Autodesk Inventor part; units mm, degrees
ref_plane "YZ Plane" through (0, 0, 0) normal (1, 0, 0) x (0, 1, 0)
ref_plane "XZ Plane" through (0, 0, 0) normal (0, 1, 0) x (-1, 0, 0)
ref_plane "XY Plane" through (0, 0, 0) normal (0, 0, 1) x (1, 0, 0)
sketch "Sketch1" plane through (0, 0, 0) normal (0, 0, 1) x (1, 0, 0)
  line L0 (0, 0) -> (45, 0)
  line L1 (45, 0) -> (45, 45)
  line L2 (45, 45) -> (0, 45)
  line L3 (0, 45) -> (0, 0)
  dimension "d0" = 45
  dimension "d1" = 45
extrude "Extrusion1" add sketch "Sketch1" along normal blind 50
fillet "Fillet1" radius 5 4 edges at (45, 45, 25) (0, 45, 25) (45, 0, 25) (0, 0, 25)
sketch "Sketch2" plane through (0, 0, 0) normal (0, 0, -1) x (-1, 0, 0)
  line L0 (-45, 5) -> (-45, 40)
  line L1 (-45, 22.5) -> (-22.5, 22.5)
  circle A0 centre (-22.5, 22.5) radius 7.5
  point P0 (0, 0)
  dimension "d5" = 22.5
  dimension "d6" = 15
extrude "Extrusion2" cut sketch "Sketch2" against normal blind 20
sketch "Sketch3" plane through (0, 0, 50) normal (0, 0, 1) x (1, 0, 0)
  line L0 (0, 0) -> (3.5, 0)
  line L1 (5, 0) -> (40, 0)
  line L2 (3.5, 0) -> (3.5, 12)
  line L3 (3.5, 12) -> (41.5, 12)
  line L4 (41.5, 12) -> (41.5, 33)
  line L5 (41.5, 33) -> (3.5, 33)
  line L6 (3.5, 33) -> (3.5, 12)
  dimension "d11" = 3.5
  dimension "d12" = 12
  dimension "d13" = 38
  dimension "d14" = 21
extrude "Extrusion3" cut sketch "Sketch3" against normal blind 12
sketch "Sketch4" plane through (0, 0, 38) normal (0, 0, 1) x (1, 0, 0)
  line L0 (3.5, 12) -> (3.5, 33)
  line L1 (3.5, 22.5) -> (29.5, 22.5)
  line L2 (29.5, 22.5) -> (33.5, 22.5)
  line L3 (3.5, 33) -> (41.5, 33)
  line L4 (30.5, 33) -> (37.7775, 33)
  line L5 (37.7775, 33) -> (37.7775, 12)
  line L6 (37.7775, 12) -> (30.5, 12)
  line L7 (30.5, 12) -> (30.5, 33)
  point P0 (0, 0)
  dimension "d20" = 26
  dimension "d21" = 4
extrude "Extrusion4" cut sketch "Sketch4" against normal blind 7 contours L3 L5 L6 L7
sketch "Sketch5" plane through (0, 0, 38) normal (0, 0, 1) x (1, 0, 0)
  circle A0 centre (9.0685, 22.5) radius 3.5
  point P0 (0, 0)
  dimension "d24" = 7
extrude "Extrusion5" cut sketch "Sketch5" against normal blind 40
sketch "Sketch6" plane through (0, 0, 50) normal (0, 0, 1) x (1, 0, 0)
  line L0 (3.5, 33) -> (30.5, 33)
  line L1 (3.5, 33) -> (0, 33)
  line L2 (0, 40) -> (0, 5)
  line L3 (3.5, 11.9982) -> (0, 11.9982)
  line L4 (0, 33) -> (3.5, 33)
  line L5 (3.5, 33) -> (3.5, 11.9982)
  line L6 (3.5, 11.9982) -> (0, 11.9982)
  line L7 (0, 11.9982) -> (0, 33)
  point P0 (0, 0)
extrude "Extrusion6" add sketch "Sketch6" along normal blind 30
fillet "Fillet2" radius 10.5 2 edges at (1.75, 33, 80) (1.75, 11.9982, 80)
sketch "Sketch7" plane through (0, 5, 0) normal (-1, 0, 0) x (0, 0, 1)
  arc A0 (80, 17.5) -> (69.5, 28) centre (69.5, 17.5) ccw
  circle A1 centre (69.5, 17.5) radius 1.5
  point P0 (0, -5)
  dimension "d30" = 3
extrude "Extrusion7" cut sketch "Sketch7" against normal blind 30
properties part number "Motor holder"
The listing builds one solid part. Answer for the finished solid, in the listing's coordinates (mm). A direction names the side the tool comes from. Round coordinates to 2 decimals unless told otherwise and drop trailing zeros. Loops run counter-clockwise (first coordinate to the right, second up) from the corner with the lowest first, then second, coordinate; pieces in that order, holes last. Notation, with made-up numbers: M 70.25,3.5 L 119.25,3.5 A18 cw 119.25,35.5 Z; hole C 21.25,13 d4. An arc over 180 degrees is marked long. Return JSON: item names as keys, results as strings.
Q1. Which of the six approach directions +Z, -Z, +X, -X, +Y, -Y give full straight-line access (tool end or side, diameter ignored) to faces 1 (the face through (34, 23, 31)), 2 (the face through (23, 23, 20)), 3 (the face through (2, 11.998, 60))?
Results list:
{"face 1": "+Z", "face 2": "-Z", "face 3": "+Z, +X, -X, -Y"}
Q2. Each of these flat-tipped pins is pushed along its axis until it touches: pin 1 Ø10 at (x, y) = (24, 9.5) entering from -Z; pin 2 Ø6 at (x, y) = (27, 5.5) entering from +Z; pin 3 Ø10.5 at (x, y) = (23.5, 27) entering from +Z; pin 4 Ø6.5 at (x, y) = (9.07, 22.5) entering from -Z. Where does it stop, or does it pass through?
Results list:
{"pin 1": "stops at z = 0", "pin 2": "stops at z = 50", "pin 3": "stops at z = 38", "pin 4": "passes through"}
Q3. Find the intervals of material crossed by line 1 along Y through (x, z) = (1.35, 69.5); line 2 along X through (y, z) = (29, 33.5); line 3 along X through (y, z) = (17.5, 47), in increasing order. Write a range as from..to.
Results list:
{"line 1": "y = 12..21, 24..33", "line 2": "x = 0..30.5, 37.78..45", "line 3": "x = 0..3.5, 41.5..45"}
Q4. Find section C-C, the plane y = 35.5. Determine the outline of the cut face in (x, z), plus the area to 3 significant figures.
Results list:
{"outline": "M 0,0 L 45,0 L 45,50 L 0,50 Z", "area": "2,250 mm2"}
Q5. Find section A-A, the plane z = 39.5. Determine the outline of the cut face in (x, y), plus the area to 3 significant figures.
Results list:
{"outline": "M 0,5 A5 ccw 5,0 L 40,0 A5 ccw 45,5 L 45,40 A5 ccw 40,45 L 5,45 A5 ccw 0,40 Z; hole M 3.5,12 L 41.5,12 L 41.5,33 L 3.5,33 Z", "area": "1,210 mm2"}
Q6. The mould has two halves that part along X. Classify faces 4 (the face through (22, 38, 50)), 5 (the face through (0, 23, 31)), 6 (the face through (23, 33, 43)): released by +X, released by -X, zero draft, split by the parting line, or undercut.
Results list:
{"face 4": "zero draft", "face 5": "released by -X", "face 6": "undercut"}
Q7. Find section D-D, the plane x = 21. Determine the outline of the cut face in (y, z).
Results list:
{"outline": "M 0,0 L 15.15,0 L 15.15,20 L 29.85,20 L 29.85,0 L 45,0 L 45,50 L 33,50 L 33,38 L 12,38 L 12,50 L 0,50 Z"}
Q8. Find section B-B, the plane x = 32. Determine the outline of the cut face in (y, z).
Results list:
{"outline": "M 0,0 L 45,0 L 45,50 L 33,50 L 33,31 L 12,31 L 12,50 L 0,50 Z"}
